For this review, take the finished solid that the model builds, in its own axes (mm). Face numbers are marked on the shaded views. A direction names the side the tool comes from. Give positions to 0.01 mm unless a question says otherwise; leave off trailing zeros. Loops run counter-clockwise (first coordinate to the right, second up) from the corner with the lowest first, then second, coordinate; pieces in that order, holes last.
```python
from build123d import *

# Parameters (mm, degrees)
EXTRUDE_1_DEPTH     = 60
CUT_EXTRUDE_1_REACH = 210.806
SKETCH_7_R          = 3.25
CUT_EXTRUDE_2_DEPTH = 5


# Read off the part's stored shape, not the designer's step: M3 すきま穴1
with BuildPart() as part:
    # ｽｹｯﾁ1 → ﾎﾞｽ - 押し出し1 (new body)
    with BuildSketch(Plane.XY):
        with BuildLine():
            Line((0, 0), (30, 120))
            Line((30, 120), (35, 120))
            ThreePointArc((35, 120), (80, 98.079568547), (125, 120))
            Line((125, 120), (130, 120))
            Line((130, 120), (160, 0))
            Line((160, 0), (0, 0))
        make_face()
    extrude(amount=EXTRUDE_1_DEPTH)

    # ｽｹｯﾁ2 → ｶｯﾄ - 押し出し1 (cut, up to next)
    with BuildSketch(Plane.XY.offset(60), mode=Mode.PRIVATE) as cut_extrude_1_sk1:
        Polygon((2.5, 10), (12.5, 10), (12.5, 50), align=None)
    cut_extrude_1_tool1 = extrude(cut_extrude_1_sk1.sketch, amount=-CUT_EXTRUDE_1_REACH, mode=Mode.PRIVATE) & part.part
    # ｽｹｯﾁ2 → ｶｯﾄ - 押し出し1 (cut, up to next)
    with BuildSketch(Plane.XY.offset(60), mode=Mode.PRIVATE) as cut_extrude_1_sk2:
        Polygon((157.5, 10), (147.5, 10), (147.5, 50), align=None)
    cut_extrude_1_tool2 = extrude(cut_extrude_1_sk2.sketch, amount=-CUT_EXTRUDE_1_REACH, mode=Mode.PRIVATE) & part.part
    add(cut_extrude_1_tool1.solids().sort_by_distance((9.166667, 23.333333, 60))[0], mode=Mode.SUBTRACT)
    add(cut_extrude_1_tool2.solids().sort_by_distance((150.833333, 23.333333, 60))[0], mode=Mode.SUBTRACT)

    # M3 すきま穴1 outline → M3 すきま穴1 (revolve, cut)
    with BuildSketch(Plane(origin=(152.5, 0, 50), x_dir=(1, 0, 0), z_dir=(0, 0, 1))):
        Polygon((0, 0), (1.7, 0), (1.7, 9.97124079), (1.725, 10), (0, 10), align=None)
    revolve(axis=Axis((152.5, 0, 50), (0, 1, 0)), mode=Mode.SUBTRACT)

    # Hole Wizard M3 _1 2 outline → Hole Wizard M3 _1 2 (revolve, cut)
    with BuildSketch(Plane(origin=(152.5, 0, 10), x_dir=(1, 0, 0), z_dir=(0, 0, 1))):
        Polygon((0, 0), (1.7, 0), (1.7, 9.97124079), (1.725, 10), (0, 10), align=None)
    revolve(axis=Axis((152.5, 0, 10), (0, 1, 0)), mode=Mode.SUBTRACT)

    # Hole Wizard M3 _1 3 outline → Hole Wizard M3 _1 3 (revolve, cut)
    with BuildSketch(Plane(origin=(7.5, 0, 50), x_dir=(1, 0, 0), z_dir=(0, 0, 1))):
        Polygon((0, 0), (1.7, 0), (1.7, 9.97124079), (1.725, 10), (0, 10), align=None)
    revolve(axis=Axis((7.5, 0, 50), (0, 1, 0)), mode=Mode.SUBTRACT)

    # Hole Wizard M3 _1 4 outline → Hole Wizard M3 _1 4 (revolve, cut)
    with BuildSketch(Plane(origin=(7.5, 0, 10), x_dir=(1, 0, 0), z_dir=(0, 0, 1))):
        Polygon((0, 0), (1.7, 0), (1.7, 9.97124079), (1.725, 10), (0, 10), align=None)
    revolve(axis=Axis((7.5, 0, 10), (0, 1, 0)), mode=Mode.SUBTRACT)

    # ｽｹｯﾁ7 → ｶｯﾄ - 押し出し2 (cut)
    with BuildSketch(Plane.XZ):
        with Locations((7.5, 50)):
            Circle(SKETCH_7_R)
        with Locations((7.5, 10)):
            Circle(SKETCH_7_R)
        with Locations((152.5, 10)):
            Circle(SKETCH_7_R)
        with Locations((152.5, 50)):
            Circle(SKETCH_7_R)
    extrude(amount=-CUT_EXTRUDE_2_DEPTH, mode=Mode.SUBTRACT)


solid = part.part
```
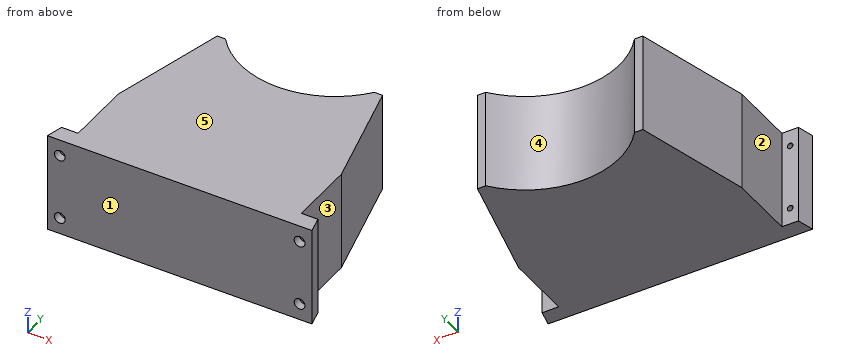
Q1. For pin 1 Ø6 at (x, z) = (70.5, 32) entering from +Y; pin 2 Ø3 at (x, z) = (8.5, 38) entering from +Y; pin 3 Ø7 at (x, z) = (152, 49) entering from -Y; pin 4 Ø3 at (y, z) = (52, 17.5) entering from -X (3 decimals), all flat-tipped, find the tip position at first contact; note any pin that passes through.
Answers:
pin 1: stops at y = 99.46
pin 2: stops at y = 10
pin 3: stops at y = 0
pin 4: stops at x = 12.625
Q2. For probe 1 along Z at (x, y) = (152.5, 1.65); probe 2 along Z at (x, y) = (152.5, 7.4); probe 3 along X at (y, z) = (7, 50), list the stretches that pass through material, from the lowest coordinate up.
Answers:
probe 1: z = 0 to 6.75, 13.25 to 46.75, 53.25 to 60
probe 2: z = 0 to 8.3, 11.7 to 48.3, 51.7 to 60
probe 3: x = 1.75 to 5.8, 9.2 to 150.8, 154.2 to 158.25
Q3. Consider section C-C on y = 38. Give the boundary of the cut face in (x, z), plus the area to 3 significant figures.
Answers:
outline: (12.5, 0) - (147.5, 0) - (147.5, 60) - (12.5, 60) - close
area: 8,100 mm2
Q4. Consider section D-D on x = 40.5. Give the boundary of the cut face in (y, z).
Answers:
outline: (0, 0) - (113.93, 0) - (113.93, 60) - (0, 60) - close
Q5. Machinability: for the marked faces 1 and 2, which of the approach directions +Z, -Z, +X, -X, +Y, -Y give a long, thin tool a straight path to every point of the face, cutting with its end or side? Answer none if there is none.
Answers:
face 1: +Z, -Z, +X, -X, -Y
face 2: +Z, -Z, -X, +Y
Q6. Consider section B-B on x = 7.5. Give the boundary of the cut face in (y, z) (3 decimals).
Answers:
outline: (0, 0) - (10, 0) - (10, 8.275) - (9.971, 8.3) - (5, 8.3) - (5, 6.75) - (0, 6.75) - close; (0, 13.25) - (5, 13.25) - (5, 11.7) - (9.971, 11.7) - (10, 11.725) - (10, 48.275) - (9.971, 48.3) - (5, 48.3) - (5, 46.75) - (0, 46.75) - close; (0, 53.25) - (5, 53.25) - (5, 51.7) - (9.971, 51.7) - (10, 51.725) - (10, 60) - (0, 60) - close
Q7. Consider section A-A on z = 10. Count the separate pieces of the cut face and the enclosed holes in it, plus the area to 3 significant figures.
Answers:
separate pieces: 3
enclosed holes: 0
area: 13,700 mm2
Q8. Mouldability with a two-part tool opening along X and no side actions: class the marked faces 3, 4 and 5 as +X half, -X half, draft (parallel to the pull), parting line (faces both ways), or undercut.
Answers:
face 3: +X half
face 4: undercut
face 5: draft
